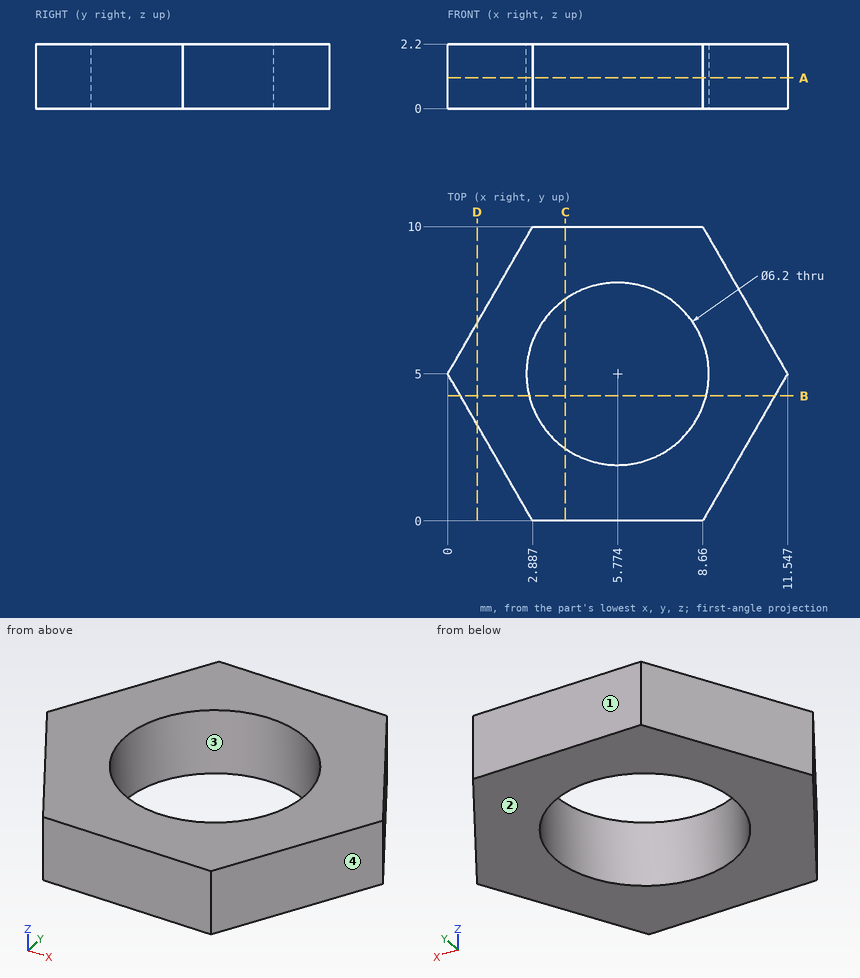
Can you work these out from the drawing? Everything is in mm from the part's minimum corner. Coordinates: 2 decimals unless noted, no trailing zeros. Loops run counter-clockwise (first coordinate to the right, second up) from the corner with the lowest first, then second, coordinate; pieces in that order, holes last.
1. Imagine slicing it at C-C, the plane x = 4. Please give me the cut outline in (y, z).
2. If we mould it in two halves opening along Y, with no side actions, what happens to the marked faces 1, 2, 3 and 4? For each: pulls with the +Y half, pulls with the -Y half, needs draft (parallel to the pull), parting line crosses it, or undercut.
3. Imagine slicing it at B-B, the plane y = 4.25. Please give me the cut outline in (x, z) (1 decimal).
4. I need wall thicknesses on L1, parallel to Y at x = 8, z = 2 (1 decimal); L2, parallel to Y at x = 3.5, z = 0.3 (1 decimal); L3, parallel to X at y = 6.5, z = 1.1 (1 decimal). Which ranges of each line are inside material? Lowest first, please.
5. Imagine slicing it at D-D, the plane x = 1. Please give me the cut outline in (y, z).
6. Imagine slicing it at A-A, the plane z = 1.05. Please give me the cut outline in (x, y).
Taken from the geometry:
1. outline: (0, 0) - (2.46, 0) - (2.46, 2.2) - (0, 2.2) - close; (7.54, 0) - (10, 0) - (10, 2.2) - (7.54, 2.2) - close
2. face 1: pulls with the +Y half
2. face 2: needs draft
2. face 3: undercut
2. face 4: pulls with the -Y half
3. outline: (0.4, 0) - (2.8, 0) - (2.8, 2.2) - (0.4, 2.2) - close; (8.8, 0) - (11.1, 0) - (11.1, 2.2) - (8.8, 2.2) - close
4. L1: y = 0 to 2.8, 7.2 to 10
4. L2: y = 0 to 2.9, 7.1 to 10
4. L3: x = 0.9 to 3.1, 8.5 to 10.7
5. outline: (3.27, 0) - (6.73, 0) - (6.73, 2.2) - (3.27, 2.2) - close
6. outline: (0, 5) - (2.89, 0) - (8.66, 0) - (11.55, 5) - (8.66, 10) - (2.89, 10) - close; hole circle Ø6.2 at (5.77, 5)
